The listing builds one solid part. Answer for the finished solid, in the listing's coordinates (mm). Face numbers are marked on the shaded views. Coordinates: 2 decimals unless noted, no trailing zeros. Order: outer loops, then holes, each group sorted by start corner. A loop starts at its lowest first (then second) coordinate and runs counter-clockwise, first axis right, second up. Notation, with made-up numbers: M 72,27 L 124,27 A34 ccw 124,59 Z; hole C -37,52.5 d3. An arc over 180 degrees is marked long. One line per item, written item: value. Start each with the question number.
Q1. Straight lines are drawn through the part: line 1 along Z through (x, y) = (0.25, -0.75); line 2 along Z through (x, y) = (1.5, -0.9); line 3 along Y through (x, z) = (1, 9). For each, find the intervals that lie inside material, in ascending order. Write a range as [from, to].
Q2. The part is cut by section C-C on z = 5.25. Give the vertices of the cut face in (x, y), then the cut area to 3 significant figures.
Q3. Determine the mould class of the marked faces 1, 2 and 3 for opening direction X: pulls with the +X half, pulls with the -X half, needs draft (parallel to the pull), parting line crosses it, or undercut.
Q4. The part is cut by section A-A on x = 0. Give the vertices of the cut face in (y, z).
Q5. Each of these flat-tipped pins is pushed along its axis until it touches: pin 1 Ø1 at (y, z) = (-1, 9.5) entering from -X; pin 2 Ø3 at (x, z) = (1.5, 9) entering from -Y; pin 3 Ø2 at (y, z) = (-1.5, 6) entering from -X. Where does it stop, or does it pass through?
Q6. The part is cut by section B-B on y = -1.3. Give the vertices of the cut face in (x, z).
Q7. The part is cut by section D-D on y = 0.8. Give the vertices of the cut face in (x, z).
```python
from build123d import *

# Parameters (mm, degrees)
SKETCH_1_R          = 1.5
EXTRUDE_1_DEPTH     = 8
SKETCH_2_R          = 3
EXTRUDE_2_DEPTH     = 0.2
DOME_1_FACE_RADIUS  = 3
DOME_1_HEIGHT       = 1.8
SKETCH_4_W          = 1.040451318
SKETCH_4_H          = 2.30386654
CUT_EXTRUDE_3_DEPTH = 50
SKETCH_7_W          = 1.027378529
SKETCH_7_H          = 1.803274818
CUT_EXTRUDE_6_DEPTH = 50


with BuildPart() as part:
    # Эскиз1 → Вытянуть1 (new body)
    with BuildSketch(Plane.XY):
        Circle(SKETCH_1_R)
    extrude(amount=EXTRUDE_1_DEPTH)

    # Эскиз2 → Вытянуть2 (add)
    with BuildSketch(Plane.XY.offset(8)):
        Circle(SKETCH_2_R)
    extrude(amount=EXTRUDE_2_DEPTH)

    # Купол1: a dome of height H over a round flat face of radius A is a cap of a sphere of radius (A * A + H * H) / (2 * H)
    dome_1_r = (DOME_1_FACE_RADIUS * DOME_1_FACE_RADIUS + DOME_1_HEIGHT * DOME_1_HEIGHT) / (2 * DOME_1_HEIGHT)
    dome_1_base = Plane((0, 0, 8.2), z_dir=(0, 0, 1))
    with Locations(dome_1_base.offset(DOME_1_HEIGHT - dome_1_r)):
        dome_1_ball = Sphere(dome_1_r, mode=Mode.PRIVATE)
    add(split(dome_1_ball, bisect_by=dome_1_base, keep=Keep.TOP, mode=Mode.PRIVATE))

    # Эскиз4 → Вырез-Вытянуть3 (cut)
    with BuildSketch(Plane(origin=(0, 0, 0), x_dir=(1, 0, 0), z_dir=(0, 1, 0))):
        with Locations((-0.049545301, -10.24795251)):
            Rectangle(SKETCH_4_W, SKETCH_4_H)
    extrude(amount=-CUT_EXTRUDE_3_DEPTH, mode=Mode.SUBTRACT)

    # Эскиз7 → Вырез-Вытянуть6 (cut)
    with BuildSketch(Plane.XZ):
        with Locations((-0.056081696, 9.997656649)):
            Rectangle(SKETCH_7_W, SKETCH_7_H)
    extrude(amount=-CUT_EXTRUDE_6_DEPTH, mode=Mode.SUBTRACT)


solid = part.part
```
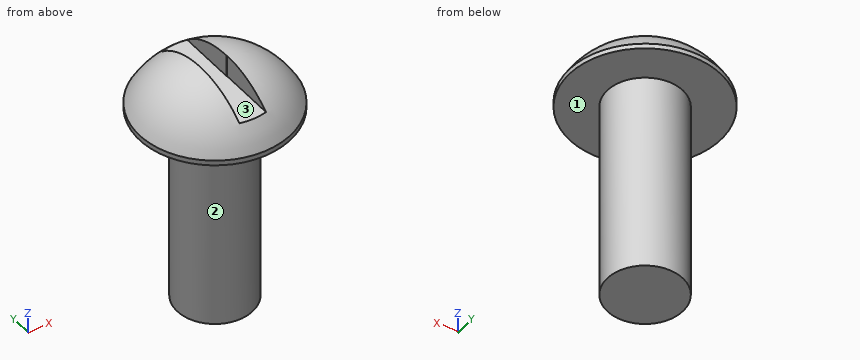
Output:
1. line 1: z = [0, 9.1]
1. line 2: z = [8, 9.52]
1. line 3: y = [-2.19, 2.19]
2. outline: C 0,0 d3
2. area: 7.07 mm^2
3. face 1: needs draft
3. face 2: parting line crosses it
3. face 3: undercut
4. outline: M -3,8 L -1.5,8 L -1.5,0 L 1.5,0 L 1.5,8 L 3,8 L 3,8.2 A3.4 ccw 2.31,9.1 L -2.31,9.1 A3.4 ccw -3,8.2 Z
5. pin 1: stops at x = -2.23
5. pin 2: stops at y = -2.99
5. pin 3: stops at x = -1.41
6. outline: M -2.7,8 L -0.75,8 L -0.75,0 L 0.75,0 L 0.75,8 L 2.7,8 L 2.7,8.2 A3.14 ccw 0.47,9.71 L 0.47,9.1 L -0.57,9.1 L -0.57,9.69 A3.14 ccw -2.7,8.2 Z
7. outline: M -2.89,8 L -1.27,8 L -1.27,0 L 1.27,0 L 1.27,8 L 2.89,8 L 2.89,8.2 A3.3 ccw 0.46,9.87 L 0.46,9.1 L -0.57,9.1 L -0.57,9.86 A3.3 ccw -2.89,8.2 Z
